Check sheet for the modelled part. Datum: model origin and axes. Units: mm. A direction names the side the tool comes from. Coordinates: 2 decimals unless noted, no trailing zeros. Write each loop counter-clockwise with the first axis right and the second up, starting at its lowest first coordinate (ties: lowest second). Pieces come first, ordered by that corner, then holes. Notation, with made-up numbers: (22, 22.5) - (43, 22.5) arc R15 ccw to (43, 46.5) - close; hole circle Ø2 at (71.25, -27). An arc over 180 degrees is marked (long way). Answer as CSV lines item,"result". Start each with the question number.
Autodesk Inventor part; units mm, degrees
ref_plane "Work Plane1" through (1.525, 0, 0) normal (0, 0, 1) x (1, 0, 0)
ref_plane "YZ Plane" through (0, 0, 0) normal (1, 0, 0) x (0, 1, 0)
ref_plane "XZ Plane" through (0, 0, 0) normal (0, 1, 0) x (-1, 0, 0)
sketch "Sketch1" plane through (0, 0, 0) normal (0, 0, 1) x (1, 0, 0)
  line L0 (0, 2.0828) -> (12.7, 2.0828)
  line L1 (12.7, 2.0828) -> (12.7, 0)
  line L2 (12.7, 0) -> (0, 0)
  line L3 (-2.54, 0) -> (15.24, 0)
  line L4 (0, -0.4166) -> (0, 2.4994)
  line L5 (0, 2.0828) -> (0, 0)
  dimension "d2" = 4.1656
  dimension "d59" = 12.7
revolve "Body" add sketch "Sketch1" angle 360 about axis through (12.7, 0, 0) along (-1, 0, 0)
sketch "Sketch2" plane through (0, 0, 0) normal (-1, 0, 0) x (0, 0, 1)
  line L0 (0, 3.6662) -> (3.175, 1.8331)
  line L1 (3.175, 1.8331) -> (3.175, -1.8331)
  line L2 (3.175, -1.8331) -> (0, -3.6662)
  line L3 (0, -3.6662) -> (-3.175, -1.8331)
  line L4 (-3.175, -1.8331) -> (-3.175, 1.8331)
  line L5 (-3.175, 1.8331) -> (0, 3.6662)
  line L6 (-4.445, 0) -> (4.445, 0)
  line L7 (0, 5.1326) -> (0, -5.1326)
  point P0 (0, 0)
  point P1 (0, 0)
  dimension "d11" = 6.35
extrude "Head" add sketch "Sketch2" along normal blind 2.794
sketch "Sketch4" plane through (0, 0, 0) normal (0, 0, 1) x (1, 0, 0)
  line L0 (-2.4274, 3.81) -> (-2.794, 3.175)
  line L1 (-1.1, 0) -> (-0.234, 0)
  line L2 (-3.306, 0) -> (0.278, 0)
  line L3 (-2.794, 3.81) -> (-2.4274, 3.81)
  line L4 (-2.794, 3.175) -> (-2.794, 3.81)
  line L5 (0, 4.572) -> (0, -0.762)
  dimension "d65" = 6.35
  dimension "d67" = 30
  dimension "d68" = 7.62
  dimension "d69" = 2.794
revolve "Chamfer1" cut sketch "Sketch4" angle 360 about axis through (-1.1, 0, 0) along (1, 0, 0)
thread "Thread"
chamfer "Chamfer2" distance 0.3975 distance2 0.3976 1 edges at (12.7, -2.0828, 0) measured on face at (12.7, 0.4208, -1.1095)
fillet "Fillet" radius 0.4166 1 edges at (0, -2.0828, 0)
ref_plane "Work Plane1" through (1.525, 0, 0) normal (0, 0, 1) x (1, 0, 0)
equation "\"d2\" = GD"
equation "\"d11\" = SW"
equation "\"d3\" = KOH"
equation "\"d15\" = GEL"
equation "\"d6\" = -0.5 * SPD + 0.5 * GD"
equation "\"d71\" = RR"
equation "\"d65\" = SW"
equation "\"d67\" = ANG1"
equation "\"d68\" = 1.2 * SW"
equation "\"d69\" = KOH"
equation "\"NLG\" = 31.75"
equation "\"GD\" = NND"
equation "\"BDM\" = NND"
equation "\"KOH\" = 2.794"
equation "\"GEL\" = 31.26232"
equation "\"SW\" = 6.35"
equation "\"SW0\" = SW"
equation "\"SPD\" = GD1"
equation "\"SD2\" = NND"
equation "\"SD\" = 0"
equation "\"ANG1\" = 30deg"
equation "\"GAL\" = 0.39751"
equation "\"GUL\" = GAL"
equation "\"RR\" = 0.41656"
equation "\"RR1\" = 0.1"
equation "\"GD1\" = 3.37058"
equation "\"THREADDIA\" = 4.1656"
equation "\"TOA\" = 30deg"
equation "\"NND\" = 4.1656"
equation "\"E0\" = 1.155 * SW"
properties part number "ANSI B18.6.3 - No. 8 - 32 - 1 1/4" material "Steel, Mild"
(1) Tool access check on faces 1 (the face through (0, 0, -3)), 2 (the face through (-1.377, -2.737, 1.61)). Record the directions out of +Z, -Z, +X, -X, +Y, -Y that give a thin tool (end or side, any length) a straight path to the whole face; none if there is none.
(2) Cross-section at A-A on x = 11.75. Record the boundary of the cut face in (y, z), plus the area to 3 significant figures.
(3) Material ranges on probe 1 along X at (y, z) = (2.25, 2); probe 2 along Y at (x, z) = (6, 0.5); probe 3 along Z at (x, y) = (1.75, -1.5), recorded low to high. Write a range as from..to.
(4) Go/stop test with flat-tipped pins: P1, Ø1, axis at x = 6.5, y = 1, coming from the -Z side; P2, Ø1, axis at x = 4, z = -2, coming from the +Y side (3 decimals); P3, Ø2, axis at x = 5, z = -2, coming from the +Y side. Record where each tip stops, or that it passes through.
Checked values:
1,face 1,"+X"
1,face 2,"+Z, +X, -X, -Y"
2,outline,"circle Ø4.17 at (0, 0)"
2,area,"13.6 mm^2"
3,probe 1,"-2.79..0"
3,probe 2,"-2.02..2.02"
3,probe 3,"-1.45..1.45"
4,P1,"z = -2.02"
4,P2,"y = 1.445"
4,P3,"y = 1.83"
